Check sheet for the drawn part. Datum: minimum x, y, z corner. Units: mm. A direction names the side the tool comes from. Coordinates: 2 decimals unless noted, no trailing zeros. Order: outer loops, then holes, each group sorted by start corner. A loop starts at its lowest first (then second) coordinate and runs counter-clockwise, first axis right, second up.
Q1. Thickness scan on line 1 (X direction, y = 10.9, z = 4); line 2 (X direction, y = 6.25, z = 6.5); line 3 (Y direction, x = 66, z = 42.5). Record the ranges inside material, lowest first.
Q2. Cross-section at C-C, the plane z = 31. Record the boundary of the cut face in (x, y), and give its area (3 significant figures).
Q3. Set-up check for the marked faces 4, 5 and 6: record each of +Z, -Z, +X, -X, +Y, -Y from which the full face is reachable in a straight line by a thin tool's end or side.
Q4. Draft check along X on the marked faces 1, 2 and 3. Enter one of: pulls with the +X half, pulls with the -X half, needs draft (parallel to the pull), parting line crosses it, or undercut.
Q5. Cross-section at D-D, the plane z = 4. Record the boundary of the cut face in (x, y).
Q6. Cross-section at A-A, the plane x = 34. Record the boundary of the cut face in (y, z).
Q7. Cross-section at B-B, the plane x = 66. Record the boundary of the cut face in (y, z), and give its area (3 significant figures).
Q8. Depth check by flat-ended pin: P1, Ø1.9, axis at x = 14, z = 4, coming from the -Y side; P2, Ø2.5, axis at y = 10.5, z = 26, coming from the -X side; P3, Ø2.5, axis at x = 2.5, y = 10.5, coming from the -Z side; P4, Ø4, axis at x = 35.5, y = 3.5, coming from the +Z side. Enter the tip coordinate at first touch or a pass-through.
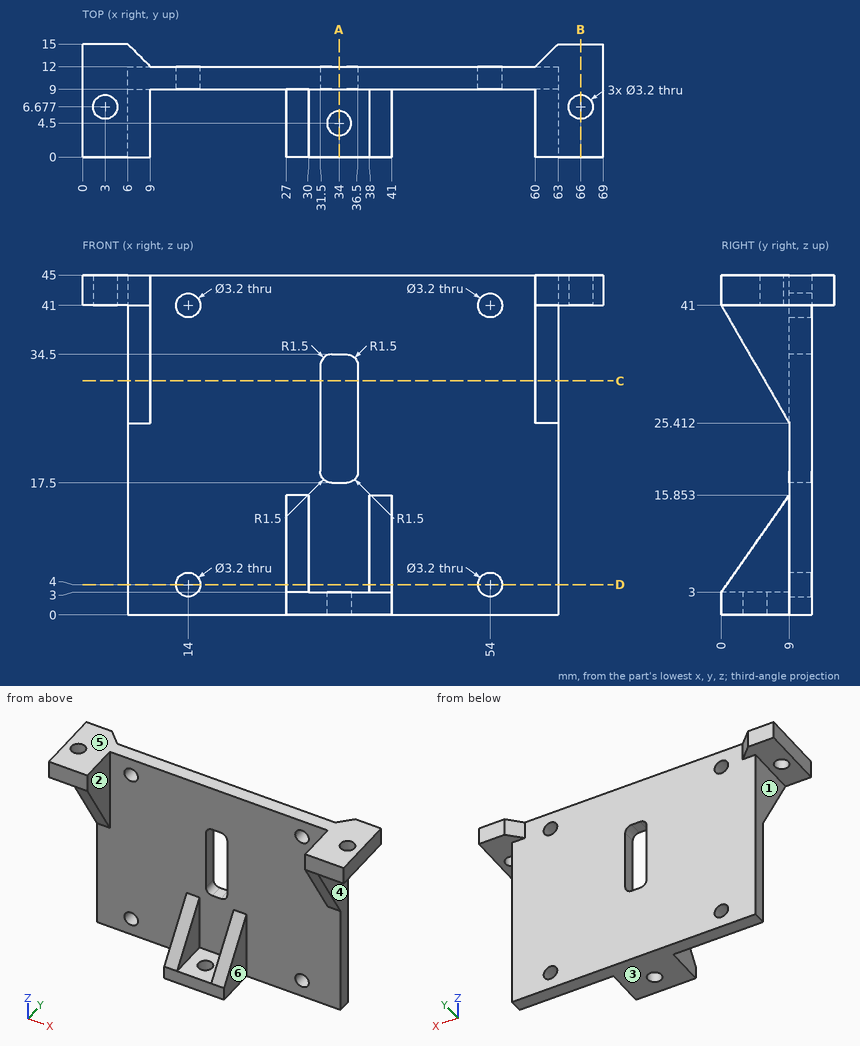
Check values:
1. line 1: x = 6 to 12.4, 15.6 to 52.4, 55.6 to 63
1. line 2: x = 27 to 30, 38 to 41
1. line 3: y = 0 to 5.08, 8.28 to 15
2. outline: (6, 5.77) - (9, 5.77) - (9, 9) - (31.5, 9) - (31.5, 12) - (6, 12) - close; (36.5, 9) - (60, 9) - (60, 5.77) - (63, 5.77) - (63, 12) - (36.5, 12) - close
2. area: 175 mm2
3. face 4: -Z, +X, +Y, -Y
3. face 5: +Z, +X, -X, +Y, -Y
3. face 6: +Z, -Z, +X, -Y
4. face 1: pulls with the -X half
4. face 2: undercut
4. face 3: needs draft
5. outline: (6, 9) - (12.4, 9) - (12.4, 12) - (6, 12) - close; (15.6, 9) - (27, 9) - (27, 0.7) - (30, 0.7) - (30, 9) - (38, 9) - (38, 0.7) - (41, 0.7) - (41, 9) - (52.4, 9) - (52.4, 12) - (15.6, 12) - close; (55.6, 9) - (63, 9) - (63, 12) - (55.6, 12) - close
6. outline: (0, 0) - (2.9, 0) - (2.9, 3) - (0, 3) - close; (6.1, 0) - (12, 0) - (12, 17.5) - (9, 17.5) - (9, 3) - (6.1, 3) - close; (9, 34.5) - (12, 34.5) - (12, 45) - (9, 45) - close
7. outline: (0, 41) - (5.08, 41) - (5.08, 45) - (0, 45) - close; (8.28, 41) - (15, 41) - (15, 45) - (8.28, 45) - close
7. area: 47.2 mm2
8. P1: passes through
8. P2: stops at x = 6
8. P3: stops at z = 41
8. P4: stops at z = 3
